Here's how the part is built. I have some questions about the finished solid (model axes, mm). A direction names the side the tool comes from. Give positions to 0.01 mm unless a question says otherwise; leave off trailing zeros. Write each loop counter-clockwise with the first axis right and the second up, starting at its lowest first coordinate (ties: lowest second). Pieces come first, ordered by that corner, then holes. Notation, with made-up numbers: (-24.5, 73) -> (28.5, 73) arc R13 cw to (28.5, 83) -> close; hole circle Ø2 at (73, -30). An arc over 180 degrees is marked (long way). Return JSON: item names as keys, results as strings.
from build123d import *

# Parameters (mm, degrees)
SKETCH1_R           = 2.1
SKETCH1_R_2         = 20
BOSS_EXTRUDE1_DEPTH = 3
FILLET1_R           = 60
FILLET3_R           = 45


with BuildPart() as part:
    # Sketch1 → Boss-Extrude1 (new body)
    with BuildSketch(Plane.XY):
        with BuildLine():
            Line((-106.261095469, -50.001427337), (-67.693838888, -95.964093924))
            Line((-67.693838888, -95.964093924), (0, -39.16221868))
            Line((0, -39.16221868), (67.693838888, -95.964093924))
            Line((67.693838888, -95.964093924), (106.261095469, -50.001427337))
            Line((106.261095469, -50.001427337), (44.97754002, 1.421581438))
            ThreePointArc((44.97754002, 1.421581438), (0, 45), (-44.97754002, 1.421581438))
            Line((-44.97754002, 1.421581438), (-106.261095469, -50.001427337))
        make_face()
        with Locations((-61.332221397, -84.099026587)):
            Circle(SKETCH1_R, mode=Mode.SUBTRACT)
        with Locations((-77.40191164, -64.947915509)):
            Circle(SKETCH1_R, mode=Mode.SUBTRACT)
        with Locations((-93.471601882, -45.796804431)):
            Circle(SKETCH1_R, mode=Mode.SUBTRACT)
        with Locations((-27.978646344, -56.112054061)):
            Circle(SKETCH1_R, mode=Mode.SUBTRACT)
        with Locations((-44.048336586, -36.960942983)):
            Circle(SKETCH1_R, mode=Mode.SUBTRACT)
        with Locations((-60.118026828, -17.809831905)):
            Circle(SKETCH1_R, mode=Mode.SUBTRACT)
        Circle(SKETCH1_R_2, mode=Mode.SUBTRACT)
        with Locations((60.118026828, -17.809831905)):
            Circle(SKETCH1_R, mode=Mode.SUBTRACT)
        with Locations((61.332221397, -84.099026587)):
            Circle(SKETCH1_R, mode=Mode.SUBTRACT)
        with Locations((77.40191164, -64.947915509)):
            Circle(SKETCH1_R, mode=Mode.SUBTRACT)
        with Locations((27.978646344, -56.112054061)):
            Circle(SKETCH1_R, mode=Mode.SUBTRACT)
        with Locations((44.048336586, -36.960942983)):
            Circle(SKETCH1_R, mode=Mode.SUBTRACT)
        with Locations((93.471601882, -45.796804431)):
            Circle(SKETCH1_R, mode=Mode.SUBTRACT)
    extrude(amount=BOSS_EXTRUDE1_DEPTH)

    # Fillet1
    fillet1_edges = [part.edges().sort_by_distance(p)[0] for p in [
        (44.97754002, 1.421581438, 1.5),
        (-44.97754002, 1.421581438, 1.5),
    ]]
    fillet(fillet1_edges, radius=FILLET1_R)

    # Fillet3
    fillet3_edges = [part.edges().sort_by_distance(p)[0] for p in [
        (0, -39.16221868, 1.5),
    ]]
    fillet(fillet3_edges, radius=FILLET3_R)


solid = part.part
1. Suppose I cut it at B-B, the plane y = 0. List the corners of the cut face in (x, z) for me, and give its area (3 significant figures).
Taken from the geometry:
{"outline": "(-49.97, 0) -> (-20, 0) -> (-20, 3) -> (-49.97, 3) -> close; (20, 0) -> (49.97, 0) -> (49.97, 3) -> (20, 3) -> close", "area": "180 mm²"}
2. Which directions (+Z, -Z, +X, -X, +Y, -Y) give clear straight access to the entire face, cutting with the end or side of a thin tool? Please do faces 1 (the face through (-60.2, -82.33, 1.48)), 2 (the face through (48.04, -79.47, 1.48)).
Taken from the geometry:
{"face 1": "+Z, -Z", "face 2": "+Z, -Z, -Y"}
3. Suppose I cut it at A-A, the plane x = 0. List the corners of the cut face in (y, z) for me, and give its area (3 significant figures).
Taken from the geometry:
{"outline": "(-52.91, 0) -> (-20, 0) -> (-20, 3) -> (-52.91, 3) -> close; (20, 0) -> (45, 0) -> (45, 3) -> (20, 3) -> close", "area": "174 mm²"}
4. If I drill on line 1 (X direction, y = 8, z = 1.85); line 2 (Y direction, x = 16.5, z = 2.2); line 3 (X direction, y = -16, z = 1.4), over which ranges is the centre line in solid material (lowest first)? Write a range as [from, to].
Taken from the geometry:
{"line 1": "x = [-45.29, -18.33], [18.33, 45.29]", "line 2": "y = [-56.04, -11.3], [11.3, 41.87]", "line 3": "x = [-65.74, -61.18], [-59.05, -12], [12, 59.05], [61.18, 65.74]"}
5. For pin 1 Ø1.5 at (x, z) = (44.5, 0.5) entering from +Y; pin 2 Ø1.5 at (y, z) = (24, 2.5) entering from +X, each with a flat end and sliding along its axis, tell me the tip position at first contact or that it passes through.
Taken from the geometry:
{"pin 1": "stops at y = 11.46", "pin 2": "stops at x = 38.53"}
6. Suppose I cut it at D-D, the plane x = 39.5. List the corners of the cut face in (y, z) for me.
Taken from the geometry:
{"outline": "(-72.31, 0) -> (21.56, 0) -> (21.56, 3) -> (-72.31, 3) -> close"}
7. If we mould it in two halves opening along X, with no side actions, what happens to faces 3 (the face through (0.781, 44.993, 1.479)), 4 (the face through (-0.44, -52.908, 1.521)), 5 (the face through (-1, -24, 3))? For each: released by +X, released by -X, zero draft, split by the parting line, or undercut.
Taken from the geometry:
{"face 3": "split by the parting line", "face 4": "undercut", "face 5": "zero draft"}
8. Suppose I cut it at C-C, the plane z = 1.4. Count the separate pieces of the cut face and the enclosed holes in it, and give its area (3 significant figures).
Taken from the geometry:
{"separate pieces": "1", "enclosed holes": "13", "area": "13,900 mm²"}
